```python
from build123d import *

# Parameters (mm, degrees)
F0_W     = 8.1
F0_H     = 3.25
F0_R     = 1.5
F0_R_2   = 4
F0_R_3   = 18
F1_DEPTH = 3


with BuildPart() as f1:
    # F0 (on Front) → F1 (new body)
    with BuildSketch(Plane.XZ):
        Polygon((-75, -14.166667), (-75, -42.5), (-25, -42.5), (-25, -39.5), (25, -39.5), (25, -42.5), (75, -42.5), (75, -14.166667), (72, -14.166667), (72, 14.166667), (75, 14.166667), (75, 42.5), (25, 42.5), (25, 39.5), (-25, 39.5), (-25, 42.5), (-75, 42.5), (-75, 14.166667), (-72, 14.166667), (-72, -14.166667), align=None)
        Polygon((-58.533333, -2.85), (-58.533333, 0), (-58.533333, 0.4), (-50.433333, 0.4), (-50.433333, -2.85), align=None, mode=Mode.SUBTRACT)
        with Locations((-6.383333, -1.225)):
            Rectangle(F0_W, F0_H, mode=Mode.SUBTRACT)
        with Locations((0, -32.2)):
            Circle(F0_R, mode=Mode.SUBTRACT)
        with Locations((0, -20.9)):
            Circle(F0_R_2, mode=Mode.SUBTRACT)
        with Locations((6.383333, -1.225)):
            Rectangle(F0_W, F0_H, mode=Mode.SUBTRACT)
        with Locations((54.483333, -1.225)):
            Rectangle(F0_W, F0_H, mode=Mode.SUBTRACT)
        with Locations((-64.7, 0)):
            Circle(F0_R, mode=Mode.SUBTRACT)
        with Locations((-30.433333, 6.9)):
            Circle(F0_R_3, mode=Mode.SUBTRACT)
        with Locations((30.433333, 6.9)):
            Circle(F0_R_3, mode=Mode.SUBTRACT)
        with Locations((64.7, 0)):
            Circle(F0_R, mode=Mode.SUBTRACT)
        with Locations((0, 32.2)):
            Circle(F0_R, mode=Mode.SUBTRACT)
    extrude(amount=F1_DEPTH)


with BuildPart() as f2_1:
    # F2: copy of F1
    add(f1.part.moved(Location((0, 60, 0))))


solid = f1.part
```
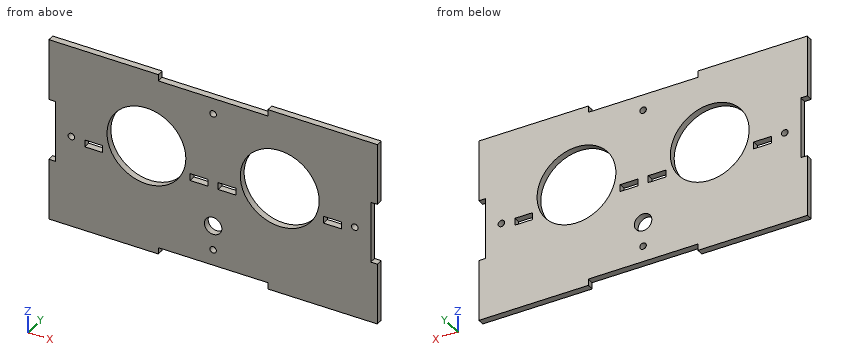
Verification items for the finished model (mm, model axes). Coordinates: 2 decimals unless noted, no trailing zeros. Loops run counter-clockwise (first coordinate to the right, second up) from the corner with the lowest first, then second, coordinate; pieces in that order, holes last. Notation, with made-up numbers: (53.5, -27.5) - (93.5, -27.5) arc R27 ccw to (93.5, 11.5) - close; hole circle Ø1 at (42, 4). An arc over 180 degrees is marked (long way). Answer as a JSON object with one key per item and string values.
(1) Go/stop test with flat-tipped pins: pin 1 Ø1.5 at (y, z) = (-2, -1.5) entering from -X; pin 2 Ø4 at (x, z) = (-64.7, 0) entering from -Y; pin 3 Ø1.5 at (y, z) = (-1.5, -1.5) entering from +X. Record where each tip stops, or that it passes through.
Response:
{"pin 1": "stops at x = -72", "pin 2": "stops at y = -3", "pin 3": "stops at x = 72"}
(2) Cross-section at B-B, the plane x = 64.7. Record the boundary of the cut face in (y, z), then the cut area to 3 significant figures.
Response:
{"outline": "(-3, -42.5) - (0, -42.5) - (0, -1.5) - (-3, -1.5) - close; (-3, 1.5) - (0, 1.5) - (0, 42.5) - (-3, 42.5) - close", "area": "246 mm²"}
(3) Cross-section at A-A, the plane z = 32.2. Record the boundary of the cut face in (x, y), then the cut area to 3 significant figures.
Response:
{"outline": "(-75, -3) - (-1.5, -3) - (-1.5, 0) - (-75, 0) - close; (1.5, -3) - (75, -3) - (75, 0) - (1.5, 0) - close", "area": "441 mm²"}
(4) Cross-section at D-D, the plane x = 0. Record the boundary of the cut face in (y, z), then the cut area to 3 significant figures.
Response:
{"outline": "(-3, -39.5) - (0, -39.5) - (0, -33.7) - (-3, -33.7) - close; (-3, -30.7) - (0, -30.7) - (0, -24.9) - (-3, -24.9) - close; (-3, -16.9) - (0, -16.9) - (0, 30.7) - (-3, 30.7) - close; (-3, 33.7) - (0, 33.7) - (0, 39.5) - (-3, 39.5) - close", "area": "195 mm²"}
(5) Scan lines: line 1 along Z through (x, y) = (0, -1.05); line 2 along Z through (x, y) = (64.7, -2.1); line 3 along Z through (x, y) = (-5, -1.05). Record each from-to range of solid material in increasing order.
Response:
{"line 1": "z = -39.5 to -33.7, -30.7 to -24.9, -16.9 to 30.7, 33.7 to 39.5", "line 2": "z = -42.5 to -1.5, 1.5 to 42.5", "line 3": "z = -39.5 to -2.85, 0.4 to 39.5"}
(6) Cross-section at C-C, the plane z = 6.9. Record the boundary of the cut face in (x, y), then the cut area to 3 significant figures.
Response:
{"outline": "(-72, -3) - (-48.43, -3) - (-48.43, 0) - (-72, 0) - close; (-12.43, -3) - (12.43, -3) - (12.43, 0) - (-12.43, 0) - close; (48.43, -3) - (72, -3) - (72, 0) - (48.43, 0) - close", "area": "216 mm²"}
